Part model, mm, in its own coordinate system. Face numbers are marked on the shaded views. A direction names the side the tool comes from. Give positions to 0.01 mm unless a question says otherwise; leave off trailing zeros. Loops run counter-clockwise (first coordinate to the right, second up) from the corner with the lowest first, then second, coordinate; pieces in that order, holes last. Notation, with made-up numbers: M 89.25,78.5 L 124.25,78.5 A27 ccw 124.25,116.5 Z; hole C 74,56 d2. An arc over 180 degrees is marked long. Answer in a Markdown table with one row per item.
from build123d import *

# Parameters (mm, degrees)
SKETCH2_R          = 4
CUT_EXTRUDE1_DEPTH = 154.785564992


with BuildPart() as part:
    # Sketch1 → Revolve1 (revolve)
    with BuildSketch(Plane.XY, mode=Mode.PRIVATE) as revolve1_sk:
        Polygon((27.5, -1.48189165), (27.5, -41.48189165), (105, -41.48189165), (105, -33.48189165), (90, -27.48189165), (90, -15.48189165), (105, -9.48189165), (105, -1.48189165), align=None)
    revolve(revolve1_sk.sketch.rotate(Axis((0, 0, 0), (0, -1, 0)), 90), axis=Axis((0, 0, 0), (0, -1, 0)))

    # Sketch2 → Cut-Extrude1 (cut, through all)
    with BuildSketch(Plane(origin=(0, -1.48189165, 0), x_dir=(1, 0, 0), z_dir=(0, 1, 0))):
        with Locations(Location((-11.379541398, -35.786671236, 0), (0, 0, 270))):
            Circle(SKETCH2_R)
        with Locations(Location((13.608078504, -35, 0), (0, 0, 270))):
            Circle(SKETCH2_R)
        with Locations(Location((14.552551693, -65, 0), (0, 0, 270))):
            Circle(SKETCH2_R)
        with Locations(Location((-10.435068209, -65.786671236, 0), (0, 0, 270))):
            Circle(SKETCH2_R)
    cut_extrude1 = extrude(amount=-CUT_EXTRUDE1_DEPTH, mode=Mode.SUBTRACT)

    # Mirror1: Cut-Extrude1 across plane
    add(cut_extrude1.mirror(Plane.XY), mode=Mode.SUBTRACT)


solid = part.part
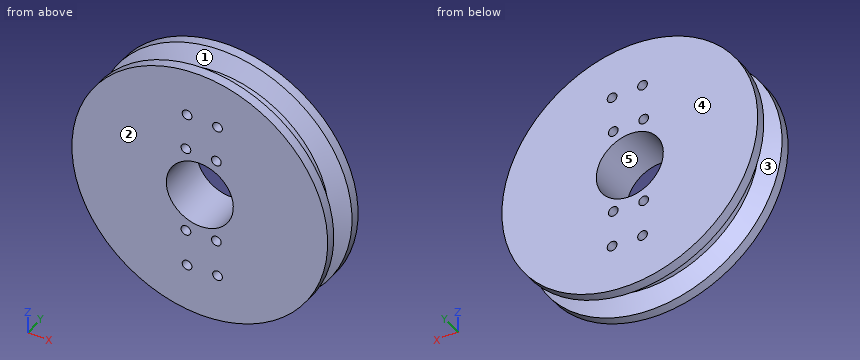
(1) Drill centre lines: line 1 along Z through (x, y) = (-0.5, -40); line 2 along X through (y, z) = (-22, 0); line 3 along X through (y, z) = (-34, -4). Where is each one in solid material? Low to high.
Recorded:
| item | result |
|---|---|
| line 1 | z = -105 to -27.5, 27.5 to 105 |
| line 2 | x = -90 to -27.5, 27.5 to 90 |
| line 3 | x = -104.92 to -27.21, 27.21 to 104.92 |
(2) Which spindle directions (+Z, -Z, +X, -X, +Y, -Y) get a long thin tool onto all of the face, cutting with end or side? Do the marked faces 1 and 2. Say none if no direction does.
Recorded:
| item | result |
|---|---|
| face 1 | none |
| face 2 | +Z, -Z, +X, -X, -Y |
(3) Pull direction Y, two halves, no side cores. Call the marked faces 3, 4 and 5: +Y half, -Y half, draft (parallel to the pull), parting line (faces both ways), or undercut.
Recorded:
| item | result |
|---|---|
| face 3 | undercut |
| face 4 | +Y half |
| face 5 | draft |
(4) Saw through at A-A (z = 0). Write the cut outline in (x, y), plus the area to 3 significant figures.
Recorded:
| item | result |
|---|---|
| outline | M -105,-41.48 L -27.5,-41.48 L -27.5,-1.48 L -105,-1.48 L -105,-9.48 L -90,-15.48 L -90,-27.48 L -105,-33.48 Z; M 27.5,-41.48 L 105,-41.48 L 105,-33.48 L 90,-27.48 L 90,-15.48 L 105,-9.48 L 105,-1.48 L 27.5,-1.48 Z |
| area | 5,660 mm^2 |
(5) Pin check, flat tips, straight feed: pin 1 Ø8 at (y, z) = (-12, 33) entering from -X; pin 2 Ø10 at (y, z) = (-8.5, -46) entering from +X; pin 3 Ø6 at (y, z) = (-9.5, 47.5) entering from -X. Stop position of each tip, or through.
Recorded:
| item | result |
|---|---|
| pin 1 | stops at x = -100.66 |
| pin 2 | stops at x = 96.66 |
| pin 3 | stops at x = -95.1 |
(6) Saw through at B-B (y = -20). Give the number of separate pieces and of enclosed holes in the cut face, plus the area to 3 significant figures.
Recorded:
| item | result |
|---|---|
| separate pieces | 1 |
| enclosed holes | 9 |
| area | 22,700 mm^2 |
